Check sheet for the modelled part. Datum: model origin and axes. Units: mm. Face numbers are marked on the shaded views. Coordinates: 2 decimals unless noted, no trailing zeros. Loops run counter-clockwise (first coordinate to the right, second up) from the corner with the lowest first, then second, coordinate; pieces in that order, holes last. Notation, with made-up numbers: (16.5, 10) - (38.5, 10) arc R25 cw to (38.5, 36) - close; hole circle Ø2 at (19.25, -37.5). An arc over 180 degrees is marked (long way). Use a Markdown table: item, result. Add a question column.
1) Sectioned sample at C-C, the plane z = -0.5. Enter the section's corners in (x, y), then the cut area to 3 significant figures.
2) Thickness scan on line 1 (X direction, y = 2.25, z = 25.25) (3 decimals); line 2 (X direction, y = 17.5, z = -11); line 3 (Z direction, x = 12.93, y = 1.7). Record the ranges inside material, lowest first.
3) Draft check along X on the marked faces 1, 2, 3 and 4. Enter one of: pulls with the +X half, pulls with the -X half, needs draft (parallel to the pull), parting line crosses it, or undercut.
4) Go/stop test with flat-tipped pins: P1, Ø3, axis at x = -29, z = 25.25, coming from the -Y side; P2, Ø1.5, axis at x = -8, y = 1, coming from the -Z side; P3, Ø2.5, axis at x = 34, y = 17.5, coming from the +Z side; P4, Ø1.5, axis at x = 3.5, z = 8, coming from the +Y side. Record where each tip stops, or that it passes through.
5) Sectioned sample at D-D, the plane y = 20.5. Enter the section's corners in (x, z), then the cut area to 3 significant figures.
6) Sectioned sample at A-A, the plane x = 12.93. Enter the section's corners in (y, z).
7) Sectioned sample at B-B, the plane y = 11. Enter the section's corners in (x, z).
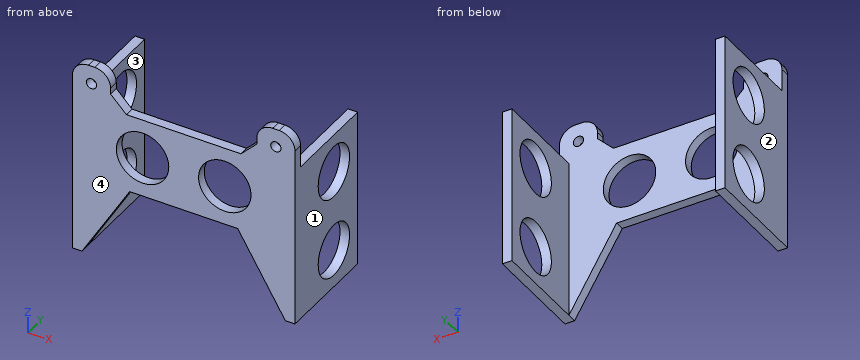
from build123d import *

# Parameters (mm, degrees)
CROQUIS1_W                 = 70
CROQUIS1_H                 = 62
SALIENTE_EXTRUIR1_DEPTH    = 3
CORTAR_EXTRUIR1_DEPTH      = 47.8508271
CORTAR_EXTRUIR2_DEPTH      = 47.8508271
CROQUIS4_W                 = 46
CROQUIS4_H                 = 10
CORTAR_EXTRUIR3_DEPTH      = 47.8508271
CROQUIS5_W                 = 46
CROQUIS5_H                 = 2
CORTAR_EXTRUIR4_DEPTH      = 47.8508271
CORTAR_EXTRUIR5_DEPTH      = 47.8508271
CORTAR_EXTRUIR5_DEPTH_BACK = 47.8508271
CROQUIS6_R                 = 1.625
CHAFL_N1_START             = -4
CHAFL_N1_OUTLINE_W         = 7.071067812
CHAFL_N1_OUTLINE_H         = 3
CHAFL_N1_DEPTH             = 4.707106781
CHAFL_N2_START             = -0.707106781
CHAFL_N2_OUTLINE_W         = 7.071067812
CHAFL_N2_OUTLINE_H         = 3
CHAFL_N2_DEPTH             = 4.707106781
CORTAR_EXTRUIR6_DEPTH      = 47.8508271
CORTAR_EXTRUIR6_DEPTH_BACK = 47.8508271
CROQUIS7_R                 = 8.25
SALIENTE_EXTRUIR2_DEPTH    = 3
CORTAR_EXTRUIR7_DEPTH      = 69.23672032
CORTAR_EXTRUIR7_DEPTH_BACK = 69.23672032
CORTAR_EXTRUIR8_DEPTH      = 47.8508271
CHAFL_N3_DEPTH             = 3
CHAFL_N5_DEPTH             = 3
CROQUIS13_W                = 50
CROQUIS13_H                = 30
SALIENTE_EXTRUIR3_DEPTH    = 3
CROQUIS14_W                = 50
CROQUIS14_H                = 30
SALIENTE_EXTRUIR4_DEPTH    = 3
REDONDEO1_R                = 5
CORTAR_EXTRUIR9_DEPTH      = 84.366660003
CORTAR_EXTRUIR9_DEPTH_BACK = 84.366660003
CROQUIS16_R                = 8.25


with BuildPart() as part:
    # Croquis1 → Saliente-Extruir1 (new body)
    with BuildSketch(Plane(origin=(0, 0, 0), x_dir=(1, 0, 0), z_dir=(0, 1, 0))):
        Rectangle(CROQUIS1_W, CROQUIS1_H)
    extrude(amount=SALIENTE_EXTRUIR1_DEPTH)

    # Croquis2 → Cortar-Extruir1 (cut, through all)
    with BuildSketch(Plane(origin=(0, 3, 0), x_dir=(1, 0, 0), z_dir=(0, 1, 0))):
        Polygon((31.754264805, 31), (15.877132403, 58.5), (-15.877132403, 58.5), (-31.754264805, 31), (-15.877132403, 3.5), (15.877132403, 3.5), align=None)
    extrude(amount=-CORTAR_EXTRUIR1_DEPTH, mode=Mode.SUBTRACT)

    # Croquis3 → Cortar-Extruir2 (cut, through all)
    with BuildSketch(Plane(origin=(0, 3, 0), x_dir=(1, 0, 0), z_dir=(0, 1, 0))):
        with BuildLine():
            Line((-13, -21), (13, -21))
            ThreePointArc((13, -21), (23, -31), (13, -41))
            Line((13, -41), (-13, -41))
            ThreePointArc((-13, -41), (-23, -31), (-13, -21))
        make_face()
    extrude(amount=-CORTAR_EXTRUIR2_DEPTH, mode=Mode.SUBTRACT)

    # Croquis4 → Cortar-Extruir3 (cut, through all)
    with BuildSketch(Plane(origin=(0, 3, 0), x_dir=(1, 0, 0), z_dir=(0, 1, 0))):
        with Locations((0, -26)):
            Rectangle(CROQUIS4_W, CROQUIS4_H)
    extrude(amount=-CORTAR_EXTRUIR3_DEPTH, mode=Mode.SUBTRACT)

    # Croquis5 → Cortar-Extruir4 (cut, through all)
    with BuildSketch(Plane(origin=(0, 3, 0), x_dir=(1, 0, 0), z_dir=(0, 1, 0))):
        with Locations((0, -20)):
            Rectangle(CROQUIS5_W, CROQUIS5_H)
    extrude(amount=-CORTAR_EXTRUIR4_DEPTH, mode=Mode.SUBTRACT)

    # Croquis6 → Cortar-Extruir5 (cut, two sides: drawn at the far end of the back side and taken through both)
    with BuildSketch(Plane(origin=(0, 3, 0), x_dir=(1, 0, 0), z_dir=(0, 1, 0)).offset(-CORTAR_EXTRUIR5_DEPTH_BACK)):
        with Locations(Location((-29, -25.25, 0), (0, 0, 270))):
            Circle(CROQUIS6_R)
        with Locations(Location((29, -25.25, 0), (0, 0, 270))):
            Circle(CROQUIS6_R)
    extrude(amount=CORTAR_EXTRUIR5_DEPTH + CORTAR_EXTRUIR5_DEPTH_BACK, mode=Mode.SUBTRACT)

    # Chaflán1: read off the stored shape, not the designer's step
    # Chaflán1 outline → Chaflán1 (add)
    with BuildSketch(Plane(origin=(0, 0, 0), x_dir=(0.7071067811865471, 0, -0.707106781186548), z_dir=(0.707106781186548, 0, 0.707106781186547)).offset(CHAFL_N1_START)):
        with Locations((-29.69848481, 1.5)):
            Rectangle(CHAFL_N1_OUTLINE_W, CHAFL_N1_OUTLINE_H)
    extrude(amount=CHAFL_N1_DEPTH)

    # Chaflán2: read off the stored shape, not the designer's step
    # Chaflán2 outline → Chaflán2 (add)
    with BuildSketch(Plane(origin=(0, 0, 0), x_dir=(0.707106781186548, 0, 0.707106781186547), z_dir=(0.707106781186547, 0, -0.707106781186548)).offset(CHAFL_N2_START)):
        with Locations((29.69848481, -1.5)):
            Rectangle(CHAFL_N2_OUTLINE_W, CHAFL_N2_OUTLINE_H)
    extrude(amount=CHAFL_N2_DEPTH)

    # Croquis7 → Cortar-Extruir6 (cut, two sides: drawn at the far end of the back side and taken through both)
    with BuildSketch(Plane(origin=(0, 3, 0), x_dir=(1, 0, 0), z_dir=(0, 1, 0)).offset(-CORTAR_EXTRUIR6_DEPTH_BACK)):
        with Locations(Location((-12.93, -6.5, 0), (0, 0, 270))):
            Circle(CROQUIS7_R)
        with Locations(Location((12.93, -6.5, 0), (0, 0, 270))):
            Circle(CROQUIS7_R)
    extrude(amount=CORTAR_EXTRUIR6_DEPTH + CORTAR_EXTRUIR6_DEPTH_BACK, mode=Mode.SUBTRACT)

    # Croquis8 → Saliente-Extruir2 (add)
    with BuildSketch(Plane(origin=(0, 3, 0), x_dir=(1, 0, 0), z_dir=(0, 1, 0))):
        Polygon((15.877132403, 3.5), (31.754264805, 31), (15.877132403, 58.5), (-15.877132403, 58.5), (-31.754264805, 31), (-15.877132403, 3.5), (0, 3.5), align=None)
    extrude(amount=-SALIENTE_EXTRUIR2_DEPTH)

    # Croquis9 → Cortar-Extruir7 (cut, two sides: drawn at the far end of the back side and taken through both)
    with BuildSketch(Plane(origin=(0, 3, 0), x_dir=(1, 0, 0), z_dir=(0, 1, 0)).offset(-CORTAR_EXTRUIR7_DEPTH_BACK)):
        Polygon((-232.018715641, 31), (-35, 31), (35, 31), (232.018715641, 31), (232.018715641, 425.037431282), (-232.018715641, 425.037431282), align=None)
    extrude(amount=CORTAR_EXTRUIR7_DEPTH + CORTAR_EXTRUIR7_DEPTH_BACK, mode=Mode.SUBTRACT)

    # Croquis10 → Cortar-Extruir8 (cut, through all)
    with BuildSketch(Plane(origin=(0, 3, 0), x_dir=(1, 0, 0), z_dir=(0, 1, 0))):
        Polygon((0, 6), (-32, 6), (-32, 31), (32, 31), (32, 6), align=None)
    extrude(amount=-CORTAR_EXTRUIR8_DEPTH, mode=Mode.SUBTRACT)

    # Chaflán3: read off the stored shape, not the designer's step
    # Chaflán3 outline → Chaflán3 (add)
    with BuildSketch(Plane(origin=(0, 0, 0), x_dir=(1, 0, 0), z_dir=(0, 1, 0))):
        Polygon((-32, 6), (-17, 6), (-32, 31), align=None)
    extrude(amount=CHAFL_N3_DEPTH)

    # Chaflán5: read off the stored shape, not the designer's step
    # Chaflán5 outline → Chaflán5 (add)
    with BuildSketch(Plane(origin=(0, 0, 0), x_dir=(1, 0, 0), z_dir=(0, 1, 0))):
        Polygon((32, 6), (32, 31), (17, 6), align=None)
    extrude(amount=CHAFL_N5_DEPTH)

    # Croquis13 → Saliente-Extruir3 (add)
    with BuildSketch(Plane.ZY.offset(35)):
        with Locations((-6, 18)):
            Rectangle(CROQUIS13_W, CROQUIS13_H)
    extrude(amount=-SALIENTE_EXTRUIR3_DEPTH)

    # Croquis14 → Saliente-Extruir4 (add)
    with BuildSketch(Plane(origin=(35, 0, 0), x_dir=(0, 0, -1), z_dir=(1, 0, 0))):
        with Locations((6, 18)):
            Rectangle(CROQUIS14_W, CROQUIS14_H)
    extrude(amount=-SALIENTE_EXTRUIR4_DEPTH)

    # Redondeo1
    redondeo1_edges = [part.edges().sort_by_distance(p)[0] for p in [
        (-23, 1.5, 31),
        (23, 1.5, 31),
        (35, 1.5, 31),
        (-35, 1.5, 31),
    ]]
    fillet(redondeo1_edges, radius=REDONDEO1_R)

    # Croquis16 → Cortar-Extruir9 (cut, two sides: drawn at the far end of the back side and taken through both)
    with BuildSketch(Plane.ZY.offset(35).offset(-CORTAR_EXTRUIR9_DEPTH_BACK)):
        with Locations((-18.93, 20.5)):
            Circle(CROQUIS16_R)
        with Locations((6.93, 20.5)):
            Circle(CROQUIS16_R)
    extrude(amount=CORTAR_EXTRUIR9_DEPTH + CORTAR_EXTRUIR9_DEPTH_BACK, mode=Mode.SUBTRACT)


solid = part.part
Solved:
| question | item | result |
|---|---|---|
| 1 | outline | (-35, 0) - (-17.3, 0) - (-17.3, 3) - (-32, 3) - (-32, 16.91) - (-35, 16.91) - close; (-35, 24.09) - (-32, 24.09) - (-32, 33) - (-35, 33) - close; (-8.56, 0) - (8.56, 0) - (8.56, 3) - (-8.56, 3) - close; (17.3, 0) - (35, 0) - (35, 16.91) - (32, 16.91) - (32, 3) - (17.3, 3) - close; (32, 24.09) - (35, 24.09) - (35, 33) - (32, 33) - close |
| 1 | area | 295 mm2 |
| 2 | line 1 | x = -35 to -30.625, -27.375 to -23, 23 to 27.375, 30.625 to 35 |
| 2 | line 2 | x = -35 to -32, 32 to 35 |
| 2 | line 3 | z = -6 to -1.75, 14.75 to 19 |
| 3 | face 1 | pulls with the +X half |
| 3 | face 2 | pulls with the -X half |
| 3 | face 3 | undercut |
| 3 | face 4 | needs draft |
| 4 | P1 | passes through |
| 4 | P2 | stops at z = -6 |
| 4 | P3 | stops at z = 19 |
| 4 | P4 | stops at y = 3 |
| 5 | outline | (-35, -31) - (-32, -31) - (-32, -27.18) - (-35, -27.18) - close; (-35, -10.68) - (-32, -10.68) - (-32, -1.32) - (-35, -1.32) - close; (-35, 15.18) - (-32, 15.18) - (-32, 19) - (-35, 19) - close; (32, -31) - (35, -31) - (35, -27.18) - (32, -27.18) - close; (32, -10.68) - (35, -10.68) - (35, -1.32) - (32, -1.32) - close; (32, 15.18) - (35, 15.18) - (35, 19) - (32, 19) - close |
| 5 | area | 102 mm2 |
| 6 | outline | (0, -6) - (3, -6) - (3, -1.75) - (0, -1.75) - close; (0, 14.75) - (3, 14.75) - (3, 19) - (0, 19) - close |
| 7 | outline | (-35, -31) - (-32, -31) - (-32, 19) - (-35, 19) - close; (32, -31) - (35, -31) - (35, 19) - (32, 19) - close |
